Build history of the part. All positions in model axes, mm. A direction names the side the tool comes from. Round coordinates to 2 decimals unless told otherwise and drop trailing zeros. Loops run counter-clockwise (first coordinate to the right, second up) from the corner with the lowest first, then second, coordinate; pieces in that order, holes last. Notation, with made-up numbers: (33.5, 17) - (72.5, 17) arc R25 ccw to (72.5, 44) - close; hole circle Ø3 at (13.5, -23.75). An arc over 180 degrees is marked (long way). One line per question, with ' | ' between items. Start each with the question number.
from build123d import *

# Parameters (mm, degrees)
SKETCH2_W           = 19
SKETCH2_H           = 19
BOSS_EXTRUDE1_DEPTH = 6
SKETCH4_R           = 4.5
BOSS_EXTRUDE2_DEPTH = 76


with BuildPart() as part:
    # Sketch2 → Boss-Extrude1 (new body)
    with BuildSketch(Plane.XY):
        Rectangle(SKETCH2_W, SKETCH2_H)
    extrude(amount=BOSS_EXTRUDE1_DEPTH)

    # Sketch4 → Boss-Extrude2 (add)
    with BuildSketch(Plane(origin=(0, 0, 0), x_dir=(-1, 0, 0), z_dir=(0, 0, -1))):
        with Locations(Location((0, 0, 0), (0, 0, 180))):  # turned: the seam where the file's is
            Circle(SKETCH4_R)
    extrude(amount=BOSS_EXTRUDE2_DEPTH)

    # Sketch6 → Revolve2 (revolve)
    with BuildSketch(Plane(origin=(0, 0, 0), x_dir=(0, 0, -1), z_dir=(1, 0, 0)), mode=Mode.PRIVATE) as revolve2_sk:
        with BuildLine():
            Line((76, 0), (76, -4.56928672))
            ThreePointArc((76, -4.56928672), (76.351816001, -2.296672068), (76.469498907, 0))
            Line((76.469498907, 0), (76, 0))
        make_face()
    revolve(revolve2_sk.sketch.rotate(Axis((0, 0, -76), (0, 0, -1)), 270), axis=Axis((0, 0, -76), (0, 0, -1)))  # turned: the seam where the file's is


solid = part.part
1) Saw through at A-A on y = 0. Write the cut outline in (x, z), and give its area (3 significant figures).
2) Saw through at D-D on x = -7.75. Write the cut outline in (y, z).
3) Saw through at C-C on z = -15. Write the cut outline in (x, y).
4) Tool access for faces 1 (the flat face through (0, 9.5, 3)), 2 (the cylindrical face through (-3.32, -3.04, -37.47)): list every direction of +Z, -Z, +X, -X, +Y, -Y with a clear straight run to the whole face (end or side of a thin tool).
5) Drop flat-ended pins along their axis: pin 1 (4 mm diameter, centred on x = 5.5, y = -2, fed in from -Z); pin 2 (10 mm diameter, centred on x = 5, y = 3.5, fed in from -Z); pin 3 (3 mm diameter, centred on x = 3, z = -34.5, fed in from +Y); pin 4 (9.5 mm diameter, centred on x = 3.5, y = 2, fed in from -Z). Give the stop position or say it passes through.
6) Wall check: line 1 (Z direction, x = -5.75, y = -2.75); line 2 (Y direction, x = -0.25, z = -17.5). Give the ranges that are in metal, low to high. Write a range as [from, to].
Answer key:
1) outline: (-9.5, 0) - (-4.5, 0) - (-4.5, -76) - (-4.57, -76) arc R22.47 ccw to (4.57, -76) - (4.5, -76) - (4.5, 0) - (9.5, 0) - (9.5, 6) - (-9.5, 6) - close | area: 801 mm²
2) outline: (-9.5, 0) - (9.5, 0) - (9.5, 6) - (-9.5, 6) - close
3) outline: circle Ø9 at (0, 0)
4) face 1: +Z, -Z, +X, -X, +Y | face 2: none
5) pin 1: z = -76.14 | pin 2: z = -76.44 | pin 3: y = 4.24 | pin 4: z = -76.47
6) line 1: [0, 6] | line 2: [-4.49, 4.49]
